Part print with two shaded views. Sizes in mm from the minimum x, y, z corner. A direction names the side the tool comes from. Give positions to 0.01 mm unless a question says otherwise; leave off trailing zeros. Order: outer loops, then holes, each group sorted by start corner. A loop starts at its lowest first (then second) coordinate and runs counter-clockwise, first axis right, second up. Notation, with made-up numbers: M 56.25,79.5 L 72.25,79.5 A19 ccw 72.25,109.5 Z; hole C 29,-34.75 d10. An arc over 180 degrees is marked long. Return JSON: item names as keys, results as strings.
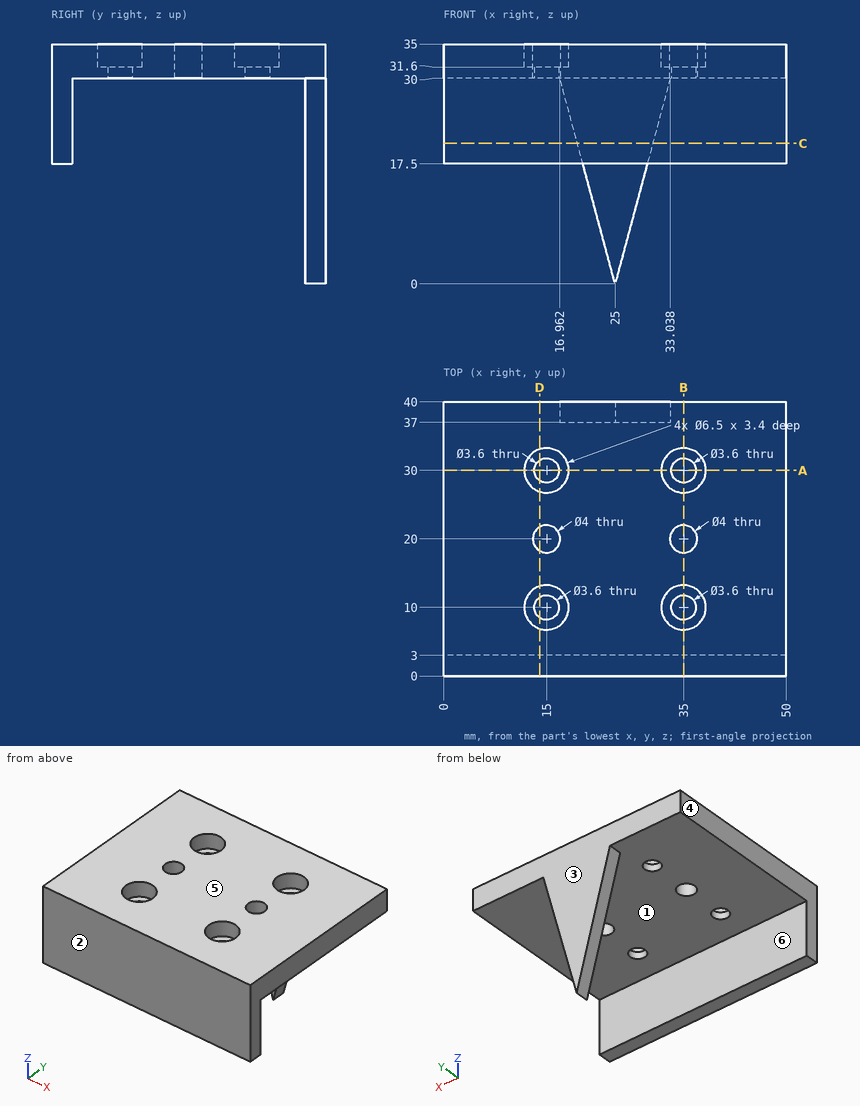
Q1. Band-saw the part on A-A (y = 30). Give the cut face in (x, z).
Established:
{"outline": "M 0,30 L 13.2,30 L 13.2,31.6 L 11.75,31.6 L 11.75,35 L 0,35 Z; M 16.8,30 L 33.2,30 L 33.2,31.6 L 31.75,31.6 L 31.75,35 L 18.25,35 L 18.25,31.6 L 16.8,31.6 Z; M 36.8,30 L 50,30 L 50,35 L 38.25,35 L 38.25,31.6 L 36.8,31.6 Z"}
Q2. Pin check, flat tips, straight feed: pin 1 (4.5 mm diameter, centred on x = 35, y = 10, fed in from -Z); pin 2 (2 mm diameter, centred on x = 38, z = 20, fed in from +Y); pin 3 (0.9 mm diameter, centred on x = 34.5, y = 2, fed in from -Z). Stop position of each tip, or through.
Established:
{"pin 1": "stops at z = 30", "pin 2": "stops at y = 3", "pin 3": "stops at z = 17.5"}
Q3. Band-saw the part on B-B (x = 35). Give the cut face in (y, z), then the cut area to 3 significant figures.
Established:
{"outline": "M 0,17.5 L 3,17.5 L 3,30 L 8.2,30 L 8.2,31.6 L 6.75,31.6 L 6.75,35 L 0,35 Z; M 11.8,30 L 18,30 L 18,35 L 13.25,35 L 13.25,31.6 L 11.8,31.6 Z; M 22,30 L 28.2,30 L 28.2,31.6 L 26.75,31.6 L 26.75,35 L 22,35 Z; M 31.8,30 L 40,30 L 40,35 L 33.25,35 L 33.25,31.6 L 31.8,31.6 Z", "area": "162 mm²"}
Q4. 3-axis set-ups, long thin cutter, end or side, ignore diameter. For the marked faces 5 and 6: which of +Z, -Z, +X, -X, +Y, -Y reach the whole face in a straight line?
Established:
{"face 5": "+Z, +X, -X, +Y, -Y", "face 6": "-Z, +X, -X"}
Q5. Probe line 1 along Y through (x, z) = (35, 33.5); line 2 along Y through (x, z) = (15, 30.7); line 3 along Z through (x, y) = (44, 27). List the from-to ranges inside material, lowest first.
Established:
{"line 1": "y = 0 to 6.75, 13.25 to 18, 22 to 26.75, 33.25 to 40", "line 2": "y = 0 to 8.2, 11.8 to 18, 22 to 28.2, 31.8 to 40", "line 3": "z = 30 to 35"}
Q6. Two-plate mould, pull along Y, no slides. Class the marked faces 1, 2, 3 and 4: +Y half, -Y half, draft (parallel to the pull), parting line (faces both ways), or undercut.
Established:
{"face 1": "undercut", "face 2": "-Y half", "face 3": "+Y half", "face 4": "draft"}
Q7. Band-saw the part on D-D (x = 14). Give the cut face in (y, z).
Established:
{"outline": "M 0,17.5 L 3,17.5 L 3,30 L 8.5,30 L 8.5,31.6 L 6.91,31.6 L 6.91,35 L 0,35 Z; M 11.5,30 L 18.27,30 L 18.27,35 L 13.09,35 L 13.09,31.6 L 11.5,31.6 Z; M 21.73,30 L 28.5,30 L 28.5,31.6 L 26.91,31.6 L 26.91,35 L 21.73,35 Z; M 31.5,30 L 40,30 L 40,35 L 33.09,35 L 33.09,31.6 L 31.5,31.6 Z"}
Q8. Band-saw the part on C-C (z = 20.5). Give the cut face in (x, y), then the cut area to 3 significant figures.
Established:
{"outline": "M 0,0 L 50,0 L 50,3 L 0,3 Z; M 19.51,37 L 30.49,37 L 30.49,40 L 19.51,40 Z", "area": "183 mm²"}
